```python
from build123d import *

# Parameters (mm, degrees)
F1_DEPTH = 12
F3_R     = 3


with BuildPart() as f1:
    # F0 (on Front) → F1 (new body)
    with BuildSketch(Plane.XZ):
        Polygon((-479.350195, -2.526657), (-629.350195, -2.526657), (-629.350195, -42.526657), (-512.566566, -42.526657), align=None)
    extrude(amount=F1_DEPTH)

    # F3
    f3_edges = [f1.edges().sort_by_distance(p)[0] for p in [
        (-554.350195, -12, -2.526657),
        (-629.350195, -12, -22.526657),
        (-570.958381, -12, -42.526657),
        (-495.958381, -12, -22.526657),
        (-554.350195, 0, -2.526657),
        (-629.350195, 0, -22.526657),
        (-570.958381, 0, -42.526657),
        (-495.958381, 0, -22.526657),
    ]]
    fillet(f3_edges, radius=F3_R)


solid = f1.part
```
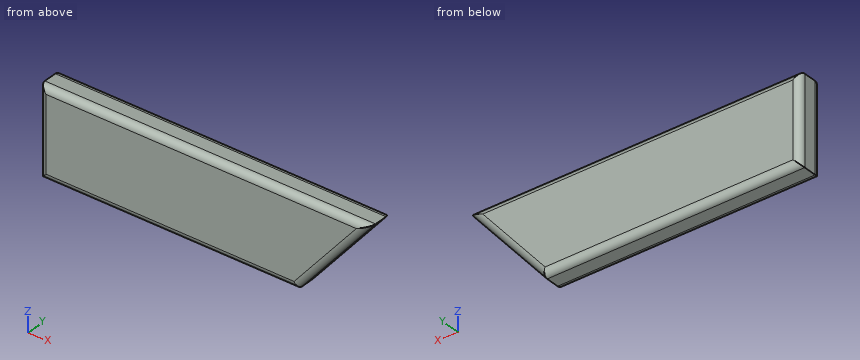
Can you work these out from the model? Positions are in its coordinate system, mm. Coordinates: 2 decimals unless noted, no trailing zeros. Loops run counter-clockwise (first coordinate to the right, second up) from the corner with the lowest first, then second, coordinate; pieces in that order, holes last. Notation, with made-up numbers: (-3, 33) - (39, 33) arc R17 ccw to (39, 39) - close; hole circle Ø7 at (-12.75, 79.5). An arc over 180 degrees is marked (long way). Use a Markdown table: item, result.
Item 1: Will this pin go through, and if not, where does the flat tip stop? pin 1 (5 mm diameter, centred on x = -497.5, y = -3.5, fed in from -Z).
Numbers:
| item | result |
|---|---|
| pin 1 | stops at z = -27.39 |
Item 2: I want a section at B-B on y = -7.5. Please give me the cut outline in (x, z), and give its area (3 significant figures).
Numbers:
| item | result |
|---|---|
| outline | (-629.35, -42.53) - (-512.57, -42.53) - (-479.35, -2.53) - (-629.35, -2.53) - close |
| area | 5,340 mm2 |
Item 3: If I drill on probe 1 along X at (y, z) = (-8.25, -20.5); probe 2 along X at (y, z) = (-8.5, -38); probe 3 along Z at (x, y) = (-564, -1), over which ranges is the centre line in solid material (lowest first)? Write a range as from..to.
Numbers:
| item | result |
|---|---|
| probe 1 | x = -629.35..-494.28 |
| probe 2 | x = -629.35..-508.81 |
| probe 3 | z = -41.76..-3.29 |
Item 4: I want a section at A-A on x = -531.5. Please give me the cut outline in (y, z), and give its area (3 significant figures).
Numbers:
| item | result |
|---|---|
| outline | (-12, -39.53) arc R3 ccw to (-9, -42.53) - (-3, -42.53) arc R3 ccw to (0, -39.53) - (0, -5.53) arc R3 ccw to (-3, -2.53) - (-9, -2.53) arc R3 ccw to (-12, -5.53) - close |
| area | 472 mm2 |
